Check sheet for the modelled part. Datum: model origin and axes. Units: mm. A direction names the side the tool comes from. Give positions to 0.01 mm unless a question says otherwise; leave off trailing zeros. Write each loop counter-clockwise with the first axis right and the second up, starting at its lowest first coordinate (ties: lowest second). Pieces come first, ordered by that corner, then holes. Notation, with made-up numbers: M 44.25,44.5 L 50.25,44.5 A7 cw 50.25,53.5 Z; hole C 79,30 d11. An arc over 180 degrees is marked long. Write item = value, one per line. Start each with the question number.
1) Gauge pin test, flat ends, axial feed: pin 1 (1 mm diameter, centred on x = -4.5, y = -0.5, fed in from -Z); pin 2 (1 mm diameter, centred on x = -1.5, y = -3, fed in from +Z); pin 3 (1 mm diameter, centred on y = 5.5, z = 4, fed in from -X). Record the tip position at first contact, or that the pin passes through.
2) Sectioned sample at B-B, the plane x = -1.75. Record the cut outline in (y, z), then the cut area to 3 significant figures.
3) Scan lines: L1, parallel to Y at x = 4.5, z = -2.75; L2, parallel to X at y = 3.75, z = 0; L3, parallel to X at y = -5.25, z = 0. Record each from-to range of solid material in increasing order.
4) Draft check along Y on faces 3 (the face through (-3, -7, 3)), 4 (the face through (1.802, -5.986, 5.723)), 5 (the face through (4.5, -5, -1.4)). Enter one of: pulls with the +Y half, pulls with the -Y half, needs draft (parallel to the pull), parting line crosses it, or undercut.
5) Sectioned sample at C-C, the plane y = -2.5. Record the cut outline in (x, z), then the cut area to 3 significant figures.
6) Set-up check for faces 1 (the face through (-2.038, 0.098, -2.658)), 2 (the face through (4.5, 5, -1.4)): record each of +Z, -Z, +X, -X, +Y, -Y from which the full face is reachable in a straight line by a thin tool's end or side.
7) Sectioned sample at D-D, the plane z = 5. Record the cut outline in (x, y).
8) Sectioned sample at A-A, the plane z = 0. Record the cut outline in (x, y).
from build123d import *

# Parameters (mm, degrees)
SKETCH1_R           = 4.5
SKETCH1_R_2         = 3.35
BOSS_EXTRUDE1_DEPTH = 5
SKETCH2_R           = 6
SKETCH2_R_2         = 3.35
BOSS_EXTRUDE2_DEPTH = 2


with BuildPart() as part:
    # Sketch1 → Boss-Extrude1 (new, symmetric)
    with BuildSketch(Plane(origin=(0, 0, 0), x_dir=(1, 0, 0), z_dir=(0, 1, 0))):
        with Locations(Location((0, 0, 0), (0, 0, 270))):
            Circle(SKETCH1_R)
        with Locations(Location((0, 0, 0), (0, 0, 270))):
            Circle(SKETCH1_R_2, mode=Mode.SUBTRACT)
    extrude(amount=BOSS_EXTRUDE1_DEPTH, both=True)

    # Sketch2 → Boss-Extrude2 (add)
    with BuildSketch(Plane(origin=(0, 5, 0), x_dir=(1, 0, 0), z_dir=(0, 1, 0))):
        with Locations(Location((0, 0, 0), (0, 0, 270))):
            Circle(SKETCH2_R)
        with Locations(Location((0, 0, 0), (0, 0, 270))):
            Circle(SKETCH2_R_2, mode=Mode.SUBTRACT)
    boss_extrude2 = extrude(amount=BOSS_EXTRUDE2_DEPTH)

    # Mirror1: Boss-Extrude2 across plane
    add(boss_extrude2.mirror(Plane.ZX))


solid = part.part
Data:
q1.pin_1 = -2.06
q1.pin_2 = 4.39
q1.pin_3 = -4.87
q2.outline = M -7,-5.74 L -5,-5.74 L -5,-4.15 L 5,-4.15 L 5,-5.74 L 7,-5.74 L 7,-2.86 L -7,-2.86 Z; M -7,2.86 L 7,2.86 L 7,5.74 L 5,5.74 L 5,4.15 L -5,4.15 L -5,5.74 L -7,5.74 Z
q2.area = 48.8 mm2
q3.L1 = -7 to -5, 5 to 7
q3.L2 = -4.5 to -3.35, 3.35 to 4.5
q3.L3 = -6 to -3.35, 3.35 to 6
q4.face_3 = pulls with the -Y half
q4.face_4 = needs draft
q4.face_5 = undercut
q5.outline = C 0,0 d9; hole C 0,0 d6.7
q5.area = 28.4 mm2
q6.face_1 = +Y, -Y
q6.face_2 = none
q7.outline = M -3.32,-7 L 3.32,-7 L 3.32,-5 L -3.32,-5 Z; M -3.32,5 L 3.32,5 L 3.32,7 L -3.32,7 Z
q8.outline = M -6,-7 L -3.35,-7 L -3.35,7 L -6,7 L -6,5 L -4.5,5 L -4.5,-5 L -6,-5 Z; M 3.35,-7 L 6,-7 L 6,-5 L 4.5,-5 L 4.5,5 L 6,5 L 6,7 L 3.35,7 Z
